Verification items for the finished model (mm, model axes). Face numbers are marked on the shaded views. A direction names the side the tool comes from. Give positions to 0.01 mm unless a question says otherwise; leave off trailing zeros. Write each loop counter-clockwise with the first axis right and the second up, starting at its lowest first coordinate (ties: lowest second). Pieces come first, ordered by that corner, then holes. Notation, with made-up numbers: M 38.5,-7 L 92.5,-7 A19 cw 92.5,-1 Z; hole C 23.5,26 d6. An arc over 180 degrees is marked long. Answer as a JSON object with one key per item and string values.
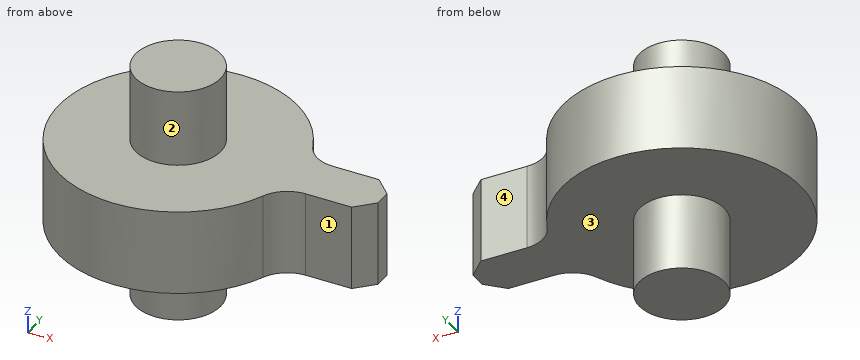
Autodesk Inventor part; units mm, degrees
ref_plane "YZ Plane" through (0, 0, 0) normal (1, 0, 0) x (0, 1, 0)
ref_plane "XZ Plane" through (0, 0, 0) normal (0, 1, 0) x (-1, 0, 0)
ref_plane "XY Plane" through (0, 0, 0) normal (0, 0, 1) x (1, 0, 0)
sketch "스케치1" plane through (0, 0, 0) normal (0, 0, 1) x (1, 0, 0)
  circle A0 centre (0, 0) radius 2.5
  arc A1 (6.8374, 1.5) -> (6.8374, -1.5) centre (0, 0) ccw
  line L0 (6.8374, 1.5) -> (12, 1.5)
  line L1 (6.8374, -1.5) -> (12, -1.5)
  line L2 (12, 1.5) -> (12, -1.5)
  dimension "d0" = 5
  dimension "d1" = 14
  dimension "d2" = 3
  dimension "d3" = 1.5
  dimension "d4" = 12
extrude "돌출1" add sketch "스케치1" along normal mid plane 5
extrude "돌출2" add sketch "스케치1" along normal mid plane 14 contours A0
chamfer "모따기1" distance 1 angle 45 2 edges at (12, 1.5, 0) (12, -1.5, 0)
fillet "모깎기1" radius 2 2 edges at (6.8374, 1.5, 0) (6.8374, -1.5, 0)
properties part number "2번부품"
1) Section check B-B on z = 0.25. Record the boundary of the cut face in (x, y), and give its area (3 significant figures).
Completed:
{"outline": "M 6.45,-2.72 A2 cw 8.29,-1.5 L 11,-1.5 L 12,-0.5 L 12,0.5 L 11,1.5 L 8.29,1.5 A2 cw 6.45,2.72 A7 ccw long Z", "area": "169 mm2"}
2) Access from +Z, -Z, +X, -X, +Y, -Y to the whole of each face (thin tool, end or side, straight path). Record for the marked faces 1, 2, 3 and 4.
Completed:
{"face 1": "+Z, -Z, +X, -Y", "face 2": "+Z", "face 3": "-Z", "face 4": "+Z, -Z, +X, +Y"}
3) Section check A-A on y = 0. Record the boundary of the cut face in (x, z).
Completed:
{"outline": "M -7,-2.5 L -2.5,-2.5 L -2.5,-7 L 2.5,-7 L 2.5,-2.5 L 12,-2.5 L 12,2.5 L 2.5,2.5 L 2.5,7 L -2.5,7 L -2.5,2.5 L -7,2.5 Z"}
4) Section check C-C on x = 0. Record the boundary of the cut face in (y, z), and give its area (3 significant figures).
Completed:
{"outline": "M -7,-2.5 L -2.5,-2.5 L -2.5,-7 L 2.5,-7 L 2.5,-2.5 L 7,-2.5 L 7,2.5 L 2.5,2.5 L 2.5,7 L -2.5,7 L -2.5,2.5 L -7,2.5 Z", "area": "115 mm2"}
5) Go/stop test with flat-tipped pins: pin 1 (4 mm diameter, centred on x = -4, z = 0, fed in from -Y); pin 2 (0.8 mm diameter, centred on x = 10.5, z = -1, fed in from -Y); pin 3 (5 mm diameter, centred on x = 10, z = 3.5, fed in from -Y). Record where each tip stops, or that it passes through.
Completed:
{"pin 1": "stops at y = -6.71", "pin 2": "stops at y = -1.5", "pin 3": "stops at y = -1.59"}
6) Thickness scan on L1, parallel to Y at x = -0.25, z = 0.5; L2, parallel to Z at x = -2.5, y = 1.75; L3, parallel to X at y = 2, z = -5. Record the ranges inside material, lowest first.
Completed:
{"L1": "y = -7 to 7", "L2": "z = -2.5 to 2.5", "L3": "x = -1.5 to 1.5"}
7) Section check D-D on y = -3. Record the boundary of the cut face in (x, z), and give its area (3 significant figures).
Completed:
{"outline": "M -6.32,-2.5 L 6.32,-2.5 L 6.32,2.5 L -6.32,2.5 Z", "area": "63.2 mm2"}
